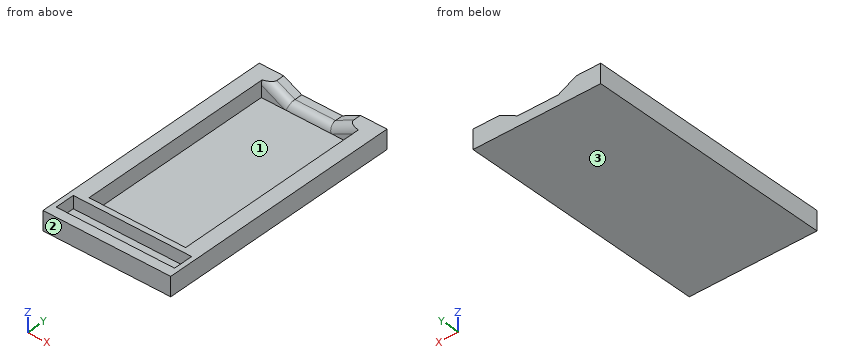
```python
from build123d import *

# Parameters (mm, degrees)
F0_W         = 82
F0_H         = 147
F0_W_2       = 62
F0_H_2       = 127
F1_DEPTH     = 12.3
F2_DEPTH     = 2
F4_DEPTH     = 12.5
F5_W         = 76
F5_H         = 12.6
F6_DEPTH     = 8
F7_DEPTH     = 25
F8_T4_DEPTH  = 38
F8_T10_DEPTH = 50.9116130734
F8_T16_DEPTH = 38
F8_T23_DEPTH = 38
F8_T28_DEPTH = 50.9116130734
F8_T35_DEPTH = 50.9116130734
F8_T39_DEPTH = 38


# Not quite as in the source:
# - a fillet or chamfer that OpenCascade refuses, or shapes differently, is made with other operations: its cross-section is extruded or revolved along the edge and cut away or added


with BuildPart() as f1:
    # F0 (on Top) → F1 (new body)
    with BuildSketch(Plane.XY):
        with Locations((0.9012136459, -11.9470648118)):
            Rectangle(F0_W, F0_H)
        with Locations((0.9012136459, -11.9470648118)):
            Rectangle(F0_W_2, F0_H_2, mode=Mode.SUBTRACT)
    extrude(amount=F1_DEPTH)

    # F0 (on Top) → F2 (join)
    with BuildSketch(Plane.XY):
        with Locations((0.9012136459, -11.9470648118)):
            Rectangle(F0_W_2, F0_H_2)
    extrude(amount=F2_DEPTH)

    # F4 (add): a face of the model
    f4_faces = [f1.faces().sort_by_distance(p)[0] for p in [
        (0.9012136459, -85.4470648118, 6.15),
    ]]
    extrude(f4_faces, amount=F4_DEPTH)

    # F5 (on face) → F6 (cut)
    with BuildSketch(Plane.XY.offset(12.3)):
        with Locations((0.9012136459, -85.3629247222)):
            Rectangle(F5_W, F5_H)
    extrude(amount=-F6_DEPTH, mode=Mode.SUBTRACT)

    # F3 (on face) → F7 (cut)
    with BuildSketch(Plane(origin=(0, 61.5529351882, 0), x_dir=(-1, 0, 0), z_dir=(0, 1, 0))):
        Polygon((24.4224453152, 12.3), (-24.8533971608, 12.3), (-13.251022455, 6.4361359849), (12.8200706095, 6.4361359849), align=None)
    extrude(amount=-F7_DEPTH, mode=Mode.SUBTRACT)

    # F8: fillet of radius 5 on 3 edges, made by hand


with BuildPart() as f8_tool2:
    # F8_s3 → F8_t4 (new body)
    with BuildSketch(Plane(origin=(-1.6465684555, 0, 0.8321790805), x_dir=(0, 1, 0), z_dir=(-0.892490362, 0, 0.4510664627))):
        with BuildLine():
            ThreePointArc((56.5529351882, 0.0385145664), (53.0174012823, 1.5029806605), (51.5529351882, 5.0385145664))
            Line((51.5529351882, 5.0385145664), (51.5529351882, 0.0385145664))
            Line((51.5529351882, 0.0385145664), (56.5529351882, 0.0385145664))
        make_face()
    extrude(amount=F8_T4_DEPTH)

    split(bisect_by=Plane.XY.offset(6.4361359849), keep=Keep.TOP)

    split(bisect_by=Plane.YZ.offset(-30.0987863541), keep=Keep.TOP)


with BuildPart() as f1_1:
    add(f1.part)

    # F8_t1: cut F8_tool2
    add(f8_tool2.part, mode=Mode.SUBTRACT)


with BuildPart() as f8_tool8:
    # F8_s9 → F8_t10 (new body)
    with BuildSketch(Plane.YZ.offset(25.6712824595)):
        with BuildLine():
            ThreePointArc((56.52103919, 6.4361359849), (53.1908229865, 5.1657016483), (51.5529351882, 2))
            Line((51.5529351882, 2), (51.5529351882, 6.4361359849))
            Line((51.5529351882, 6.4361359849), (56.52103919, 6.4361359849))
        make_face()
    extrude(amount=-F8_T10_DEPTH)

    split(bisect_by=Plane(origin=(-0.0173726292, 0, -0.0343738793), x_dir=(0, 1, 0), z_dir=(0.4510664627, 0, 0.892490362)), keep=Keep.TOP)

    split(bisect_by=Plane(origin=(0.1050545028, 0, -0.2078632285), x_dir=(0, 1, 0), z_dir=(-0.4510664627, 0, 0.892490362)), keep=Keep.TOP)


with BuildPart() as f1_2:
    add(f1_1.part)

    # F8_t7: cut F8_tool8
    add(f8_tool8.part, mode=Mode.SUBTRACT)


with BuildPart() as f8_tool14:
    # F8_s15 → F8_t16 (new body)
    with BuildSketch(Plane(origin=(35.9044721827, 0, 18.1461940123), x_dir=(0, 1, 0), z_dir=(-0.892490362, 0, -0.4510664627))):
        with BuildLine():
            ThreePointArc((56.5529351882, 0.232902491), (53.0174012823, 1.6973685851), (51.5529351882, 5.232902491))
            Line((51.5529351882, 5.232902491), (51.5529351882, 0.232902491))
            Line((51.5529351882, 0.232902491), (56.5529351882, 0.232902491))
        make_face()
    extrude(amount=F8_T16_DEPTH)

    split(bisect_by=Plane.XY.offset(6.4361359849), keep=Keep.TOP)

    split(bisect_by=Plane.YZ.offset(31.9012136459), keep=Keep.BOTTOM)


with BuildPart() as f1_3:
    add(f1_2.part)

    # F8_t13: cut F8_tool14
    add(f8_tool14.part, mode=Mode.SUBTRACT)


with BuildPart() as f8_tool21:
    # F8_s22 → F8_t23 (new body)
    with BuildSketch(Plane(origin=(-1.6465684555, 0, 0.8321790805), x_dir=(0, 1, 0), z_dir=(-0.892490362, 0, 0.4510664627))):
        with BuildLine():
            ThreePointArc((56.5529351882, 0.0385145664), (53.0174012823, 1.5029806605), (51.5529351882, 5.0385145664))
            Line((51.5529351882, 5.0385145664), (51.5529351882, 0.0385145664))
            Line((51.5529351882, 0.0385145664), (56.5529351882, 0.0385145664))
        make_face()
    extrude(amount=F8_T23_DEPTH)

    split(bisect_by=Plane.XY.offset(6.4361359849), keep=Keep.BOTTOM)

    split(bisect_by=Plane.XY.offset(2), keep=Keep.TOP)


with BuildPart() as f8_tool26:
    # F8_s27 → F8_t28 (new body)
    with BuildSketch(Plane.YZ.offset(25.6712824595)):
        with BuildLine():
            ThreePointArc((56.52103919, 6.4361359849), (53.1908229865, 5.1657016483), (51.5529351882, 2))
            Line((51.5529351882, 2), (51.5529351882, 6.4361359849))
            Line((51.5529351882, 6.4361359849), (56.52103919, 6.4361359849))
        make_face()
    extrude(amount=-F8_T28_DEPTH)

    split(bisect_by=Plane(origin=(-0.0173726292, 0, -0.0343738793), x_dir=(0, 1, 0), z_dir=(-0.4510664627, 0, -0.892490362)), keep=Keep.TOP)


with BuildPart() as f8_tool21_1:
    add(f8_tool21.part)

    # F8_t30: intersect F8_tool26
    add(f8_tool26.part, mode=Mode.INTERSECT)


with BuildPart() as f1_4:
    add(f1_3.part)

    # F8_t19: cut F8_tool21
    add(f8_tool21_1.part, mode=Mode.SUBTRACT)


with BuildPart() as f8_tool33:
    # F8_s34 → F8_t35 (new body)
    with BuildSketch(Plane.YZ.offset(25.6712824595)):
        with BuildLine():
            ThreePointArc((56.52103919, 6.4361359849), (53.1908229865, 5.1657016483), (51.5529351882, 2))
            Line((51.5529351882, 2), (51.5529351882, 6.4361359849))
            Line((51.5529351882, 6.4361359849), (56.52103919, 6.4361359849))
        make_face()
    extrude(amount=-F8_T35_DEPTH)

    split(bisect_by=Plane(origin=(0.1050545028, 0, -0.2078632285), x_dir=(0, 1, 0), z_dir=(0.4510664627, 0, -0.892490362)), keep=Keep.TOP)


with BuildPart() as f8_tool37:
    # F8_s38 → F8_t39 (new body)
    with BuildSketch(Plane(origin=(35.9044721827, 0, 18.1461940123), x_dir=(0, 1, 0), z_dir=(-0.892490362, 0, -0.4510664627))):
        with BuildLine():
            ThreePointArc((56.5529351882, 0.232902491), (53.0174012823, 1.6973685851), (51.5529351882, 5.232902491))
            Line((51.5529351882, 5.232902491), (51.5529351882, 0.232902491))
            Line((51.5529351882, 0.232902491), (56.5529351882, 0.232902491))
        make_face()
    extrude(amount=F8_T39_DEPTH)

    split(bisect_by=Plane.XY.offset(6.4361359849), keep=Keep.BOTTOM)

    split(bisect_by=Plane.XY.offset(2), keep=Keep.TOP)


with BuildPart() as f8_tool33_1:
    add(f8_tool33.part)

    # F8_t42: intersect F8_tool37
    add(f8_tool37.part, mode=Mode.INTERSECT)


with BuildPart() as f1_5:
    add(f1_4.part)

    # F8_t31: cut F8_tool33
    add(f8_tool33_1.part, mode=Mode.SUBTRACT)


solid = f1_5.part
```
Input: part model. Units: mm. Frame: model coordinates. Face numbers are marked on the shaded views. Give positions to 0.01 mm unless a question says otherwise; leave off trailing zeros. Loops run counter-clockwise (first coordinate to the right, second up) from the corner with the lowest first, then second, coordinate; pieces in that order, holes last. Notation, with made-up numbers: (1.5, 9) -> (33.5, 9) arc R9 ccw to (33.5, 24) -> close; hole circle Ø10 at (13.25, 24). An arc over 180 degrees is marked (long way). Use a Markdown table: item, result.
Q1. Section query C-C, the plane y = -33.5. Return the cut outline in (x, z), plus the area to 3 significant figures.
Entries:
| item | result |
|---|---|
| outline | (-40.1, 0) -> (41.9, 0) -> (41.9, 12.3) -> (31.9, 12.3) -> (31.9, 2) -> (-30.1, 2) -> (-30.1, 12.3) -> (-40.1, 12.3) -> close |
| area | 370 mm² |
Q2. Ray query, probe 1 along Y at (x, z) = (27, 2.25); probe 2 along Y at (x, z) = (-20.5, 11); probe 3 along X at (y, z) = (-10, 4.5). Return the intervals inside material, ascending. Write a range as from..to.
Entries:
| item | result |
|---|---|
| probe 1 | y = -97.95..-75.45, 51.55..61.55 |
| probe 2 | y = -97.95..-91.66, -79.06..-75.45 |
| probe 3 | x = -40.1..-30.1, 31.9..41.9 |
Q3. Section query B-B, the plane y = -82.5. Return the cut outline in (x, z), plus the area to 3 significant figures.
Entries:
| item | result |
|---|---|
| outline | (-40.1, 0) -> (41.9, 0) -> (41.9, 12.3) -> (38.9, 12.3) -> (38.9, 4.3) -> (-37.1, 4.3) -> (-37.1, 12.3) -> (-40.1, 12.3) -> close |
| area | 401 mm² |
Q4. Section query A-A, the plane x = 4. Return the cut outline in (y, z), plus the area to 3 significant figures.
Entries:
| item | result |
|---|---|
| outline | (-97.95, 0) -> (61.55, 0) -> (61.55, 6.44) -> (56.52, 6.44) arc R5 ccw to (51.55, 2) -> (-75.45, 2) -> (-75.45, 12.3) -> (-79.06, 12.3) -> (-79.06, 4.3) -> (-91.66, 4.3) -> (-91.66, 12.3) -> (-97.95, 12.3) -> close |
| area | 489 mm² |
Q5. First-contact query: P1, Ø6.5, axis at x = 17.5, y = -83, coming from the +Z side; P2, Ø1.5, axis at x = 18.5, y = 29, coming from the +Z side; P3, Ø2.5, axis at x = -11, z = 10, coming from the +Y side. Flat tips, straight axial feed; report the tip coordinate or a pass-through.
Entries:
| item | result |
|---|---|
| P1 | stops at z = 4.3 |
| P2 | stops at z = 2 |
| P3 | stops at y = -75.45 |
Q6. Pull-direction query (Y, two-part tool) for the marked faces 1, 2 and 3; classes: pulls with the +Y half, pulls with the -Y half, needs draft (parallel to the pull), parting line crosses it, or undercut.
Entries:
| item | result |
|---|---|
| face 1 | undercut |
| face 2 | pulls with the -Y half |
| face 3 | needs draft |
